from build123d import *

# Parameters (mm, degrees)
CHAMFER_1_SIZE      = 1
FILLET_1_R          = 1
CUT_EXTRUDE_1_DEPTH = 7


with BuildPart() as part:
    # Эскиз1 → Повернуть1 (revolve)
    with BuildSketch(Plane.XY, mode=Mode.PRIVATE) as revolve_1_sk:
        Polygon((10, 2.9), (10, 7), (8, 7), (8, 5), (0, 5), (0, 2.9), align=None)
    revolve(revolve_1_sk.sketch.rotate(Axis((0, 0, 0), (1, 0, 0)), 90), axis=Axis((0, 0, 0), (1, 0, 0)))

    # Фаска1
    chamfer_1_edges = [part.edges().sort_by_distance(p)[0] for p in [
        (0, 0, -5),
    ]]
    chamfer(chamfer_1_edges, length=CHAMFER_1_SIZE)

    # Скругление1
    fillet_1_edges = [part.edges().sort_by_distance(p)[0] for p in [
        (10, 0, -7),
        (8, 0, -7),
    ]]
    fillet(fillet_1_edges, radius=FILLET_1_R - 0.0001)  # a hair under: the kernel refuses the full size

    # Эскиз2 → Вырез-Вытянуть1 (cut)
    with BuildSketch(Plane.ZY):
        Polygon((-6, -0.5), (-0.399521329, -0.5), (-0.399521329, -5.986683782), (0.399521329, -5.986683782), (0.399521329, -0.5), (6, -0.5), (6, 0.5), (0.399521329, 0.5), (0.399521329, 5.986683782), (-0.399521329, 5.986683782), (-0.399521329, 0.5), (-6, 0.5), align=None)
    extrude(amount=-CUT_EXTRUDE_1_DEPTH, mode=Mode.SUBTRACT)


solid = part.part
The model under review builds one solid part; all positions refer to its coordinate system, in mm. A direction names the side the tool comes from. Round coordinates to 2 decimals unless told otherwise and drop trailing zeros. Loops run counter-clockwise (first coordinate to the right, second up) from the corner with the lowest first, then second, coordinate; pieces in that order, holes last. Notation, with made-up numbers: (-36, -27.5) -> (16, -27.5) arc R25 cw to (16, 7.5) -> close; hole circle Ø8 at (76.5, -28.75). An arc over 180 degrees is marked (long way). Write item = value, one per line. Start each with the question number.
Item 1: For faces 1 (the flat face through (0, 2.2, 2.2)), 2 (the flat face through (3, 4, -0.4)), 3 (the conical face through (0.27, 3.08, 2.96)), 4 (the flat face through (3, -0.5, 4)), 5 (the cylindrical face through (4.45, -1.5, 4.77)), list the 3-axis set-ups (+Z, -Z, +X, -X, +Y, -Y) from which the entire face can be reached by the end or side of a thin tool; tool diameter is ignored.
Item 2: To check wall thickness, follow L1, parallel to Y at x = 7.5, z = 0; L2, parallel to Z at x = 3.75, y = -3; L3, parallel to X at y = 2.75, z = 4.75. State the ranges of each line that lie inside material, in increasing order.
Item 3: Insertion check: pin 1 (0.6 mm diameter, centred on x = 4, z = 4.5, fed in from +Y); pin 2 (1.7 mm diameter, centred on x = 4.5, z = 4.5, fed in from -Y); pin 3 (1.7 mm diameter, centred on x = 2, y = -4.5, fed in from -Z). Each pin has a flat end and moves straight along its axis. Give the tip position at first contact, or say it passes through.
Item 4: Mouldability with a two-part tool opening along Z and no side actions: class faces 6 (the flat face through (7, 0, 4)), 7 (the flat face through (3, -4, 0.4)), 8 (the conical face through (0.27, -3.08, -2.96)) as released by +Z, released by -Z, zero draft, split by the parting line, or undercut.
Item 5: Take a section at B-B on x = 5.5. Give the boundary of the cut face in (y, z).
Result:
q1.face_1 = +Z, -Z, -X, +Y, -Y
q1.face_2 = -X, +Y, -Y
q1.face_3 = +Z, -X, +Y
q1.face_4 = +Z, -Z, -X
q1.face_5 = -X
q2.L1 = -5 to -2.9, 2.9 to 5
q2.L2 = -4 to -0.4, 0.4 to 4
q2.L3 = 8 to 10
q3.pin_1 = 2.71
q3.pin_2 = -3.42
q3.pin_3 = -3.42
q4.face_6 = zero draft
q4.face_7 = undercut
q4.face_8 = released by -Z
q5.outline = (-4.98, -0.4) arc R5 ccw to (-0.5, -4.97) -> (-0.5, -2.86) arc R2.9 cw to (-2.87, -0.4) -> close; (-4.98, 0.4) -> (-2.87, 0.4) arc R2.9 cw to (-0.5, 2.86) -> (-0.5, 4.97) arc R5 ccw to start; (0.5, -4.97) arc R5 ccw to (4.98, -0.4) -> (2.87, -0.4) arc R2.9 cw to (0.5, -2.86) -> close; (0.5, 2.86) arc R2.9 cw to (2.87, 0.4) -> (4.98, 0.4) arc R5 ccw to (0.5, 4.97) -> close
